Could you check a few things on this drawing? It's one solid part, dimensions in mm from its lowest x, y, z. A direction names the side the tool comes from. Coordinates: 2 decimals unless noted, no trailing zeros. Order: outer loops, then holes, each group sorted by start corner. A loop starts at its lowest first (then second) coordinate and runs counter-clockwise, first axis right, second up. Notation, with made-up numbers: (6, 60) -> (52, 60) arc R21 ccw to (52, 95) -> close; hole circle Ø5 at (20.25, 16.25). An arc over 180 degrees is marked (long way). Use a Markdown table: item, result. Add a question column.
1. Suppose I cut it at B-B, the plane x = 8.75. List the corners of the cut face in (y, z) for me.
2. For the marked faces 1 and 2, which set-ups out of +Z, -Z, +X, -X, +Y, -Y let a thin tool reach every point of the face, with its end or its side?
3. Suppose I cut it at D-D, the plane z = 38. List the corners of the cut face in (x, y) for me, then the cut area to 3 significant figures.
4. Suppose I cut it at A-A, the plane z = 51.5. List the corners of the cut face in (x, y) for me.
5. For pin 1 Ø6 at (x, z) = (10.5, 39) entering from -Y; pin 2 Ø0.5 at (y, z) = (11, 50) entering from -X (1 decimal); pin 3 Ø0.9 at (y, z) = (11, 53) entering from +X, each with a flat end and sliding along its axis, tell me the tip position at first contact or that it passes through.
6. If I drill on line 1 along Z through (x, y) = (8.25, 0.5); line 2 along X through (y, z) = (6.5, 46); line 3 along Y through (x, z) = (4.5, 17), over which ranges is the centre line in solid material (lowest first)? Write a range as from..to.
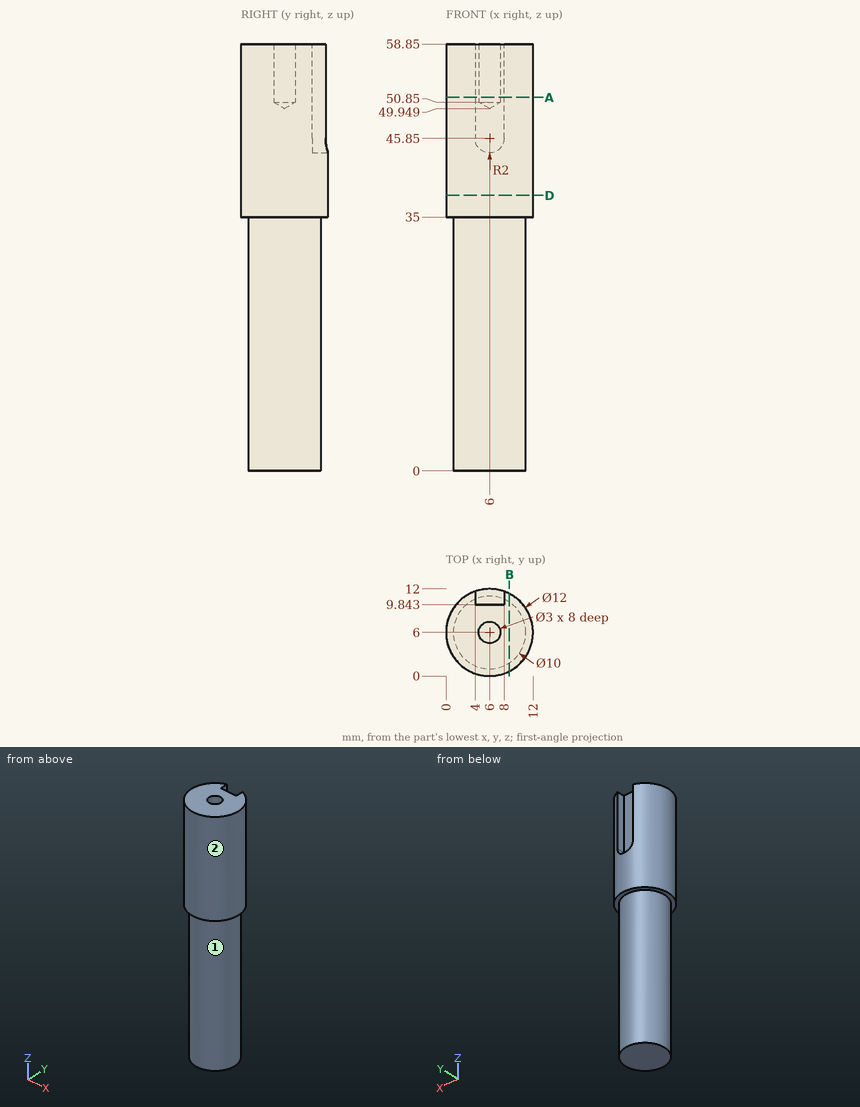
Worked out:
| question | item | result |
|---|---|---|
| 1 | outline | (0.67, 35) -> (1.82, 35) -> (1.82, 0) -> (10.18, 0) -> (10.18, 35) -> (11.33, 35) -> (11.33, 58.85) -> (0.67, 58.85) -> close |
| 2 | face 1 | -Z |
| 2 | face 2 | +Z, -Z |
| 3 | outline | circle Ø12 at (6, 6) |
| 3 | area | 113 mm² |
| 4 | outline | (4, 9.84) -> (4, 11.66) arc R6 ccw (long way) to (8, 11.66) -> (8, 9.84) -> close; hole circle Ø3 at (6, 6) |
| 5 | pin 1 | stops at y = 0.19 |
| 5 | pin 2 | stops at x = 2.3 |
| 5 | pin 3 | stops at x = 9.91 |
| 6 | line 1 | z = 35..58.85 |
| 6 | line 2 | x = 0.02..11.98 |
| 6 | line 3 | y = 1.23..10.77 |
